```python
from build123d import *

# Parameters (mm, degrees)
SKETCH1_W           = 6.35
SKETCH1_H           = 50.8
BOSS_EXTRUDE1_DEPTH = 26
SKETCH4_R           = 1.6
CUT_EXTRUDE3_DEPTH  = 6.35
SKETCH14_R          = 1.25
CUT_EXTRUDE13_DEPTH = 5
CHAMFER3_SIZE       = 0.25


with BuildPart() as part:
    # Sketch1 → Boss-Extrude1 (new body)
    with BuildSketch(Plane.XY):
        with Locations((3.175, 25.4)):
            Rectangle(SKETCH1_W, SKETCH1_H)
    extrude(amount=BOSS_EXTRUDE1_DEPTH)

    # Sketch4 → Cut-Extrude3 (cut)
    with BuildSketch(Plane(origin=(6.35, 0, 0), x_dir=(0, 0, -1), z_dir=(1, 0, 0))):
        with Locations((-3, 3.175)):
            Circle(SKETCH4_R)
        with Locations((-23, 3.175)):
            Circle(SKETCH4_R)
        with Locations((-13, 3.175)):
            Circle(SKETCH4_R)
    extrude(amount=-CUT_EXTRUDE3_DEPTH, mode=Mode.SUBTRACT)

    # Sketch14 → Cut-Extrude13 (cut)
    with BuildSketch(Plane(origin=(0, 50.8, 0), x_dir=(1, 0, 0), z_dir=(0, 1, 0))):
        with Locations(Location((3.175, -23, 0), (0, 0, 270))):
            Circle(SKETCH14_R)
        with Locations(Location((3.175, -13, 0), (0, 0, 270))):
            Circle(SKETCH14_R)
        with Locations(Location((3.175, -3, 0), (0, 0, 270))):
            Circle(SKETCH14_R)
    extrude(amount=-CUT_EXTRUDE13_DEPTH, mode=Mode.SUBTRACT)

    # Chamfer3
    chamfer3_edges = [part.edges().sort_by_distance(p)[0] for p in [
        (3.175, 50.8, 21.75),
        (3.175, 50.8, 11.75),
        (3.175, 50.8, 1.75),
    ]]
    chamfer(chamfer3_edges, length=CHAMFER3_SIZE)


solid = part.part
```
Build history of the part. All positions in model axes, mm. A direction names the side the tool comes from. Coordinates: 2 decimals unless noted, no trailing zeros. Write each loop counter-clockwise with the first axis right and the second up, starting at its lowest first coordinate (ties: lowest second). Pieces come first, ordered by that corner, then holes.
1. Band-saw the part on A-A, the plane z = 3. Give the cut face in (x, y) (3 decimals).
Answer block:
outline: (0, 0) - (6.35, 0) - (6.35, 1.575) - (0, 1.575) - close; (0, 4.775) - (6.35, 4.775) - (6.35, 50.8) - (4.675, 50.8) - (4.425, 50.55) - (4.425, 45.8) - (1.925, 45.8) - (1.925, 50.55) - (1.675, 50.8) - (0, 50.8) - close
2. Drill centre lines: probe 1 along Y at (x, z) = (5.75, 4); probe 2 along Y at (x, z) = (4.75, 23) (3 decimals); probe 3 along X at (y, z) = (49.2, 3) (3 decimals). Where is each one in solid material? Low to high.
Answer block:
probe 1: y = 0 to 1.93, 4.42 to 50.8
probe 2: y = 0 to 1.575, 4.775 to 50.8
probe 3: x = 0 to 1.925, 4.425 to 6.35
3. Band-saw the part on B-B, the plane y = 47. Give the cut face in (x, z) (3 decimals), and give its area (3 significant figures).
Answer block:
outline: (0, 0) - (6.35, 0) - (6.35, 26) - (0, 26) - close; hole circle Ø2.5 at (3.175, 3); hole circle Ø2.5 at (3.175, 13); hole circle Ø2.5 at (3.175, 23)
area: 150 mm2
4. Band-saw the part on C-C, the plane x = 5.5. Give the cut face in (y, z) (3 decimals).
Answer block:
outline: (0, 0) - (50.8, 0) - (50.8, 26) - (0, 26) - close; hole circle Ø3.2 at (3.175, 3); hole circle Ø3.2 at (3.175, 13); hole circle Ø3.2 at (3.175, 23)
5. Pull direction Y, two halves, no side cores. Call faces 1 (the cylindrical face through (4.02, 48.21, 12.08)), 2 (the flat face through (3, 0, 13)), 3 (the flat face through (3, 45.8, 23)), 4 (the cylindrical face through (3.219, 3.656, 21.474)): released by +Y, released by -Y, zero draft, split by the parting line, or undercut.
Answer block:
face 1: zero draft
face 2: released by -Y
face 3: released by +Y
face 4: undercut
6. 3-axis set-ups, long thin cutter, end or side, ignore diameter. For faces 5 (the flat face through (3, 26, 0)), 6 (the flat face through (3, 45.8, 13)): which of +Z, -Z, +X, -X, +Y, -Y reach the whole face in a straight line?
Answer block:
face 5: -Z, +X, -X, +Y, -Y
face 6: +Y
